```python
from build123d import *

# Parameters (mm, degrees)
SKETCH2_W           = 100
SKETCH2_H           = 100
SKETCH2_R           = 4
BOSS_EXTRUDE1_DEPTH = 15
SKETCH3_R           = 2.5
CUT_EXTRUDE1_DEPTH  = 15


with BuildPart() as part:
    # Sketch2 → Boss-Extrude1 (new body)
    with BuildSketch(Plane(origin=(0, 0, 0), x_dir=(0, 0, -1), z_dir=(1, 0, 0))):
        Rectangle(SKETCH2_W, SKETCH2_H)
        Circle(SKETCH2_R, mode=Mode.SUBTRACT)
    extrude(amount=BOSS_EXTRUDE1_DEPTH)

    # Sketch3 → Cut-Extrude1 (cut)
    with BuildSketch(Plane(origin=(15, 0, 0), x_dir=(0, 0, -1), z_dir=(1, 0, 0))):
        with Locations((-19.445436483, 19.445436483)):
            Circle(SKETCH3_R)
        with Locations((19.445436483, 19.445436483)):
            Circle(SKETCH3_R)
        with Locations((19.445436483, -19.445436483)):
            Circle(SKETCH3_R)
        with Locations((-19.445436483, -19.445436483)):
            Circle(SKETCH3_R)
    extrude(amount=-CUT_EXTRUDE1_DEPTH, mode=Mode.SUBTRACT)


solid = part.part
```
Check sheet for the modelled part. Datum: model origin and axes. Units: mm. Round coordinates to 2 decimals unless told otherwise and drop trailing zeros. Loops run counter-clockwise (first coordinate to the right, second up) from the corner with the lowest first, then second, coordinate; pieces in that order, holes last. Notation, with made-up numbers: (19.5, 69.25) - (78.5, 69.25) arc R31 cw to (78.5, 96.25) - close; hole circle Ø10 at (-30.75, 71.25). An arc over 180 degrees is marked (long way). Write item = value, one per line. Start each with the question number.
Q1. Depth check by flat-ended pin: P1, Ø4, axis at y = -19.45, z = -19.45, coming from the +X side. Enter the tip coordinate at first touch or a pass-through.
Q2. Thickness scan on L1, parallel to Z at x = 5, y = 17.5; L2, parallel to Z at x = 8.5, y = 2.5; L3, parallel to Y at x = 8.25, z = 0.5. Record the ranges inside material, lowest first.
Q3. Section check A-A (z = 0). Record the boundary of the cut face in (x, y), plus the area to 3 significant figures.
Q4. Release check for a two-part mould opening along Y. For faces 1 (the face through (15, 12, 1)), 2 (the face through (7, -50, 1)), 3 (the face through (7.6, -18.69, -21.83)) record: pulls with the +Y half, pulls with the -Y half, needs draft (parallel to the pull), parting line crosses it, or undercut.
Derived:
q1.P1 = through
q2.L1 = -50 to -21.02, -17.88 to 17.88, 21.02 to 50
q2.L2 = -50 to -3.12, 3.12 to 50
q2.L3 = -50 to -3.97, 3.97 to 50
q3.outline = (0, -50) - (15, -50) - (15, -4) - (0, -4) - close; (0, 4) - (15, 4) - (15, 50) - (0, 50) - close
q3.area = 1,380 mm^2
q4.face_1 = needs draft
q4.face_2 = pulls with the -Y half
q4.face_3 = undercut
